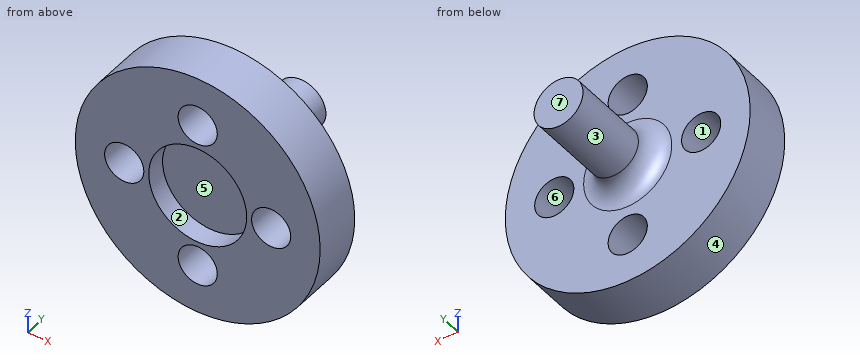
from build123d import *

# Parameters (mm, degrees)
SKETCH1_R           = 12.5
SKETCH1_R_2         = 2
BOSS_EXTRUDE1_DEPTH = 5
SKETCH2_R           = 2.5
BOSS_EXTRUDE2_DEPTH = 10
SKETCH3_R           = 5
CUT_EXTRUDE1_DEPTH  = 2
FILLET2_R           = 2


with BuildPart() as part:
    # Sketch1 → Boss-Extrude1 (new body)
    with BuildSketch(Plane(origin=(0, 0, 0), x_dir=(1, 0, 0), z_dir=(0, 1, 0))):
        Circle(SKETCH1_R)
        with Locations((-7.5, 0)):
            Circle(SKETCH1_R_2, mode=Mode.SUBTRACT)
        with Locations((0, 7.5)):
            Circle(SKETCH1_R_2, mode=Mode.SUBTRACT)
        with Locations((7.5, 0)):
            Circle(SKETCH1_R_2, mode=Mode.SUBTRACT)
        with Locations((0, -7.5)):
            Circle(SKETCH1_R_2, mode=Mode.SUBTRACT)
    extrude(amount=BOSS_EXTRUDE1_DEPTH)

    # Sketch2 → Boss-Extrude2 (add)
    with BuildSketch(Plane(origin=(0, 5, 0), x_dir=(1, 0, 0), z_dir=(0, 1, 0))):
        Circle(SKETCH2_R)
    extrude(amount=BOSS_EXTRUDE2_DEPTH)

    # Sketch3 → Cut-Extrude1 (cut)
    with BuildSketch(Plane.XZ):
        Circle(SKETCH3_R)
    extrude(amount=-CUT_EXTRUDE1_DEPTH, mode=Mode.SUBTRACT)

    # Fillet2
    fillet2_edges = [part.edges().sort_by_distance(p)[0] for p in [
        (-2.5, 5, 0),
    ]]
    fillet(fillet2_edges, radius=FILLET2_R)


solid = part.part
The listing builds one solid part. Answer for the finished solid, in the listing's coordinates (mm). Face numbers are marked on the shaded views. A direction names the side the tool comes from. Round coordinates to 2 decimals unless told otherwise and drop trailing zeros. Order: outer loops, then holes, each group sorted by start corner. A loop starts at its lowest first (then second) coordinate and runs counter-clockwise, first axis right, second up. Notation, with made-up numbers: (52, 19.25) -> (108, 19.25) arc R5 ccw to (108, 26.25) -> close; hole circle Ø1 at (-35, -18.5). An arc over 180 degrees is marked (long way). Write each question's results on one line, items separated by ' | '. Start each with the question number.
Q1. Find section B-B (x = -8.25). Determine the outline of the cut face in (y, z), then the cut area to 3 significant figures.
Q2. Straight lines are drawn through the part: probe 1 along Z at (x, y) = (0, 0.9); probe 2 along Y at (x, z) = (-10.75, 5); probe 3 along Z at (x, y) = (-0.25, 3.5). For each, find the intervals that lie inside material, in ascending order. Write a range as from..to.
Q3. Find section A-A (z = 7.5). Determine the outline of the cut face in (x, y).
Q4. Each of these flat-tipped pins is pushed along its axis until it touches: pin 1 (2 mm diameter, centred on y = 7.5, z = 0, fed in from -X); pin 2 (1 mm diameter, centred on x = -2, z = -7, fed in from +Y); pin 3 (1.5 mm diameter, centred on x = -6.5, z = 1.5, fed in from -Y); pin 4 (1.5 mm diameter, centred on y = 8, z = -3, fed in from -X). Where does it stop, or does it pass through?
Q5. Which of the six approach directions +Z, -Z, +X, -X, +Y, -Y give full straight-line access (tool end or side, diameter ignored) to the marked faces 1, 2 and 3?
Q6. Find section D-D (x = 0). Determine the outline of the cut face in (y, z), then the cut area to 3 significant figures.
Q7. Find section C-C (z = 0). Determine the outline of the cut face in (x, y), then the cut area to 3 significant figures.
Q8. The mould has two halves that part along Z. Classify the marked faces 4, 5, 6 and 7: pulls with the +Z half, pulls with the -Z half, needs draft (parallel to the pull), parting line crosses it, or undercut.
Worked answers:
1) outline: (0, -9.39) -> (5, -9.39) -> (5, -1.85) -> (0, -1.85) -> close; (0, 1.85) -> (5, 1.85) -> (5, 9.39) -> (0, 9.39) -> close | area: 75.4 mm2
2) probe 1: z = -12.5..-9.5, -5.5..-5, 5..5.5, 9.5..12.5 | probe 2: y = 0..5 | probe 3: z = -12.5..-9.48, -5.52..5.52, 9.48..12.5
3) outline: (-10, 0) -> (-2, 0) -> (-2, 5) -> (-10, 5) -> close; (2, 0) -> (10, 0) -> (10, 5) -> (2, 5) -> close
4) pin 1: stops at x = -2.56 | pin 2: stops at y = 5 | pin 3: stops at y = 0 | pin 4: stops at x = -1.09
5) face 1: +Y, -Y | face 2: -Y | face 3: +Y
6) outline: (0, -12.5) -> (5, -12.5) -> (5, -9.5) -> (0, -9.5) -> close; (0, -5.5) -> (5, -5.5) -> (5, -4.5) arc R2 cw to (7, -2.5) -> (15, -2.5) -> (15, 2.5) -> (7, 2.5) arc R2 cw to (5, 4.5) -> (5, 5.5) -> (0, 5.5) -> (0, 5) -> (2, 5) -> (2, -5) -> (0, -5) -> close; (0, 9.5) -> (5, 9.5) -> (5, 12.5) -> (0, 12.5) -> close | area: 117 mm2
7) outline: (-12.5, 0) -> (-9.5, 0) -> (-9.5, 5) -> (-12.5, 5) -> close; (-5.5, 0) -> (-5, 0) -> (-5, 2) -> (5, 2) -> (5, 0) -> (5.5, 0) -> (5.5, 5) -> (4.5, 5) arc R2 cw to (2.5, 7) -> (2.5, 15) -> (-2.5, 15) -> (-2.5, 7) arc R2 cw to (-4.5, 5) -> (-5.5, 5) -> close; (9.5, 0) -> (12.5, 0) -> (12.5, 5) -> (9.5, 5) -> close | area: 117 mm2
8) face 4: parting line crosses it | face 5: undercut | face 6: undercut | face 7: needs draft
